from build123d import *

# Parameters (mm, degrees)
F0_R     = 3.5
F0_R_2   = 1.925
F1_DEPTH = 3.9
F2_DEPTH = 35
F4_DEPTH = 2
F5_R     = 0.25


with BuildPart() as f1:
    # F0 (on Front) → F1 (new body)
    with BuildSketch(Plane.XZ):
        Circle(F0_R)
        Circle(F0_R_2, mode=Mode.SUBTRACT)
        Circle(F0_R_2)
    extrude(amount=F1_DEPTH)

    # F0 (on Front) → F2 (join)
    with BuildSketch(Plane.XZ):
        Circle(F0_R_2)
    extrude(amount=-F2_DEPTH)

    # F3 (on face) → F4 (cut)
    with BuildSketch(Plane.XZ.offset(3.9)):
        Polygon((1.5, -0.8660254038), (1.5, 0.8660254038), (0, 1.7320508076), (-1.5, 0.8660254038), (-1.5, -0.8660254038), (0, -1.7320508076), align=None)
    extrude(amount=-F4_DEPTH, mode=Mode.SUBTRACT)

    # F5
    f5_edges = [f1.edges().sort_by_distance(p)[0] for p in [
        (-3.5, -3.9, 0),
    ]]
    fillet(f5_edges, radius=F5_R)


solid = f1.part
Geometry: final body of the model. Coordinates: model frame, mm. A direction names the side the tool comes from. Coordinates: 2 decimals unless noted, no trailing zeros. Order: outer loops, then holes, each group sorted by start corner. A loop starts at its lowest first (then second) coordinate and runs counter-clockwise, first axis right, second up. Notation, with made-up numbers: (61, -6) - (86, -6) arc R28 cw to (86, 26) - close; hole circle Ø10 at (-37.5, 36). An arc over 180 degrees is marked (long way). Use one line per item in the form item = value.
1) Section B-B (y = 21.5). Return loops of the section in (x, z) (3 decimals), then the cut area to 3 significant figures.
Solutions:
outline = circle Ø3.85 at (0, 0)
area = 11.6 mm^2
2) Ray query, L1, parallel to Y at x = -0.25, z = -1.5; L2, parallel to Y at x = 2, z = 1.75; L3, parallel to Z at x = 0, y = 12.5 (3 decimals). Return the intervals inside material, ascending.
Solutions:
L1 = -1.9 to 35
L2 = -3.9 to 0
L3 = -1.925 to 1.925
3) Pin query (flat end, axial travel): pin 1 (1.5 mm diameter, centred on y = 30, z = -1, fed in from +X); pin 2 (3 mm diameter, centred on y = 2, z = 0, fed in from -X) (3 decimals); pin 3 (1 mm diameter, centred on y = 3.5, z = -2.5, fed in from +X); pin 4 (2 mm diameter, centred on x = 0, z = 0.5, fed in from -Y). Return the tip coordinate at first contact, or that it passes through.
Solutions:
pin_1 = 1.91
pin_2 = -1.925
pin_3 = through
pin_4 = -1.9
4) Section A-A (z = 0). Return loops of the section in (x, y) (3 decimals).
Solutions:
outline = (-3.5, -3.65) arc R0.25 ccw to (-3.25, -3.9) - (-1.5, -3.9) - (-1.5, -1.9) - (1.5, -1.9) - (1.5, -3.9) - (3.25, -3.9) arc R0.25 ccw to (3.5, -3.65) - (3.5, 0) - (1.925, 0) - (1.925, 35) - (-1.925, 35) - (-1.925, 0) - (-3.5, 0) - close
5) Mould query, pull axis Z, two halves, no side actions, for faces 4 (the face through (0.74, -2.914, -1.305)), 5 (the face through (0, -1.9, 0)), 6 (the face through (-0.8, -3.9, 1.5)), 7 (the face through (-0.42, 17.26, -1.88)). Classes: +Z half, -Z half, draft (parallel to the pull), parting line (faces both ways), or undercut.
Solutions:
face_4 = undercut
face_5 = undercut
face_6 = draft
face_7 = parting line
6) Set-up query: faces 1 (the face through (2, 0, -2)), 2 (the face through (0, 35, 0)), 3 (the face through (1.5, -3, 0)). Return all of +Z, -Z, +X, -X, +Y, -Y with unobstructed straight access to the full face (end or side cutting, diameter ignored); none if empty.
Solutions:
face_1 = +Y
face_2 = +Z, -Z, +X, -X, +Y
face_3 = -Y
